from build123d import *

# Parameters (mm, degrees)
F0_R     = 42
F2_DEPTH = 3
F1_R     = 40.25
F3_DEPTH = 16
F4_SIZE  = 1
F5_W     = 7
F5_H     = 3
F6_DEPTH = 50


with BuildPart() as f2:
    # F0 (on Top) → F2 (new body)
    with BuildSketch(Plane.XY):
        Circle(F0_R)
    extrude(amount=F2_DEPTH)

    # F1 (on Top) → F3 (cut)
    with BuildSketch(Plane.XY):
        Circle(F1_R)
    extrude(amount=F3_DEPTH, mode=Mode.SUBTRACT)

    # F4
    f4_edges = [f2.edges().sort_by_distance(p)[0] for p in [
        (-40.25, 0, 0),
        (-42, 0, 3),
    ]]
    chamfer(f4_edges, length=F4_SIZE)

    # F5 (on Front) → F6 (cut)
    with BuildSketch(Plane.XZ):
        with Locations((-3.5, 13.5)):
            Rectangle(F5_W, F5_H)
    extrude(amount=-F6_DEPTH, mode=Mode.SUBTRACT)


solid = f2.part
Verification items for the finished model (mm, model axes). Coordinates: 2 decimals unless noted, no trailing zeros. Write each loop counter-clockwise with the first axis right and the second up, starting at its lowest first coordinate (ties: lowest second). Pieces come first, ordered by that corner, then holes. Notation, with made-up numbers: M -33.75,43 L 6.25,43 A25 ccw 6.25,59 Z; hole C 45.5,63.5 d7. An arc over 180 degrees is marked long. Use a Markdown table: item, result.
Q1. Go/stop test with flat-tipped pins: P1, Ø1.5, axis at y = 1.5, z = 2.5, coming from the -X side; P2, Ø1, axis at y = 22.5, z = 1, coming from the -X side. Record where each tip stops, or that it passes through.
Reply:
| item | result |
|---|---|
| P1 | stops at x = -41.99 |
| P2 | stops at x = -35.78 |
Q2. Sectioned sample at A-A, the plane x = 0. Record the boundary of the cut face in (y, z).
Reply:
| item | result |
|---|---|
| outline | M -42,0 L -41.25,0 L -40.25,1 L -40.25,3 L -41,3 L -42,2 Z; M 40.25,1 L 41.25,0 L 42,0 L 42,2 L 41,3 L 40.25,3 Z |
Q3. Draft check along X on faces 1 (the face through (28, -31, 0)), 2 (the face through (40.06, 12.62, 0.99)), 3 (the face through (-40.21, 1.77, 1.99)). Enter one of: +X half, -X half, draft (parallel to the pull), parting line (faces both ways), or undercut.
Reply:
| item | result |
|---|---|
| face 1 | draft |
| face 2 | parting line |
| face 3 | undercut |
Q4. Thickness scan on line 1 (Y direction, x = 0, z = 1.95); line 2 (X direction, y = -29.5, z = 0.8); line 3 (Y direction, x = 0, z = 2.4). Record the ranges inside material, lowest first.
Reply:
| item | result |
|---|---|
| line 1 | y = -42 to -40.25, 40.25 to 42 |
| line 2 | x = -29.9 to -27.68, 27.68 to 29.9 |
| line 3 | y = -41.6 to -40.25, 40.25 to 41.6 |
